Source: CAD feature listing. Evaluate the final solid. Frame: model axes, mm. Coordinates: 2 decimals unless noted, no trailing zeros. Order: outer loops, then holes, each group sorted by start corner. A loop starts at its lowest first (then second) coordinate and runs counter-clockwise, first axis right, second up. Notation, with made-up numbers: (48.25, 25) -> (81.25, 25) arc R12 ccw to (81.25, 33) -> close; hole circle Ø11 at (78, -16). An arc over 180 degrees is marked (long way). Put each result on its own line as item: value.
from build123d import *

# Parameters (mm, degrees)
F0_W     = 101.6
F0_H     = 25.4
F0_R     = 3.175
F1_DEPTH = 3.81
F2_R     = 1.27
F3_R     = 5.08


with BuildPart() as f1:
    # F0 (on Top) → F1 (new body)
    with BuildSketch(Plane.XY):
        Rectangle(F0_W, F0_H)
        with BuildLine():
            ThreePointArc((-35.1064285714, 2.3568262774), (-22.86, 0), (-35.1064285714, -2.3568262774))
            ThreePointArc((-35.1064285714, -2.3568262774), (-41.91, 0), (-35.1064285714, 2.3568262774))
        make_face(mode=Mode.SUBTRACT)
        with Locations((-12.7, 0)):
            Circle(F0_R, mode=Mode.SUBTRACT)
        with Locations((12.7, 0)):
            Circle(F0_R, mode=Mode.SUBTRACT)
        with BuildLine():
            ThreePointArc((35.1064285714, -2.3568262774), (22.86, 0), (35.1064285714, 2.3568262774))
            ThreePointArc((35.1064285714, 2.3568262774), (41.91, 0), (35.1064285714, -2.3568262774))
        make_face(mode=Mode.SUBTRACT)
    extrude(amount=F1_DEPTH)

    # F2
    f2_edges = [f1.edges().sort_by_distance(p)[0] for p in [
        (-35.106429, -2.356826, 1.905),
        (35.106429, 2.356826, 1.905),
        (-35.106429, 2.356826, 1.905),
        (35.106429, -2.356826, 1.905),
    ]]
    fillet(f2_edges, radius=F2_R)

    # F3
    f3_edges = [f1.edges().sort_by_distance(p)[0] for p in [
        (-50.8, 12.7, 1.905),
        (-50.8, -12.7, 1.905),
        (50.8, -12.7, 1.905),
        (50.8, 12.7, 1.905),
    ]]
    fillet(f3_edges, radius=F3_R)


solid = f1.part
1. Pull-direction query (X, two-part tool) for faces 1 (the cylindrical face through (-49.351, 11.172, 1.932)), 2 (the flat face through (50.8, 0, 2)), 3 (the cylindrical face through (22.864, -0.225, 1.878)); classes: pulls with the +X half, pulls with the -X half, needs draft (parallel to the pull), parting line crosses it, or undercut.
Numbers:
face 1: pulls with the -X half
face 2: pulls with the +X half
face 3: undercut
2. Cut plane B-B on y = 5. Output: boundary loops of the cut face in (x, z).
Numbers:
outline: (-50.8, 0) -> (-33.12, 0) -> (-33.12, 3.81) -> (-50.8, 3.81) -> close; (-25.3, 0) -> (25.3, 0) -> (25.3, 3.81) -> (-25.3, 3.81) -> close; (33.12, 0) -> (50.8, 0) -> (50.8, 3.81) -> (33.12, 3.81) -> close
3. Cut plane A-A on x = 38.1. Output: boundary loops of the cut face in (y, z).
Numbers:
outline: (-12.7, 0) -> (-3.81, 0) -> (-3.81, 3.81) -> (-12.7, 3.81) -> close; (3.81, 0) -> (12.7, 0) -> (12.7, 3.81) -> (3.81, 3.81) -> close
4. Cut plane D-D on z = 2.3. Count the separate pieces of the cut face and the enclosed holes in it, plus the area to 3 significant figures.
Numbers:
separate pieces: 1
enclosed holes: 4
area: 2,160 mm2
5. Ray query, line 1 along X through (y, z) = (5.5, 2.35); line 2 along Y through (x, z) = (-29.21, 1.5); line 3 along Y through (x, z) = (-12.5, 0.4). Return the intervals inside material, ascending.
Numbers:
line 1: x = -50.8 to -32.38, -26.04 to 26.04, 32.38 to 50.8
line 2: y = -12.7 to -6.35, 6.35 to 12.7
line 3: y = -12.7 to -3.17, 3.17 to 12.7
6. Cut plane C-C on x = 12.7. Output: boundary loops of the cut face in (y, z) (3 decimals).
Numbers:
outline: (-12.7, 0) -> (-3.175, 0) -> (-3.175, 3.81) -> (-12.7, 3.81) -> close; (3.175, 0) -> (12.7, 0) -> (12.7, 3.81) -> (3.175, 3.81) -> close
7. First-contact query: pin 1 (1.5 mm diameter, centred on y = -10, z = 2.5, fed in from -X); pin 2 (1.5 mm diameter, centred on y = 10, z = 3.5, fed in from +X). Flat tips, straight axial feed; report the tip coordinate or a pass-through.
Numbers:
pin 1: stops at x = -50.53
pin 2: stops at x = 50.53
